```python
from build123d import *

# Parameters (mm, degrees)
SKETCH2_W               = 50.8
SKETCH2_H               = 50.8
BOSS_EXTRUDE1_DEPTH     = 4.7625
SKETCH3_W               = 3.175
SKETCH3_H               = 50.8
CUT_EXTRUDE1_DEPTH      = 1.5875
BOSS_EXTRUDE2_DEPTH     = 6.35
BOSS_EXTRUDE3_DEPTH     = 12.7
SKETCH6_W               = 22.225
SKETCH6_H               = 6.35
CUT_EXTRUDE2_DEPTH      = 44.45
SKETCH7_R               = 2.413
SKETCH7_R_2             = 2.286
CUT_EXTRUDE3_DEPTH      = 50.8
CUT_EXTRUDE4_DEPTH      = 3.175
CUT_EXTRUDE4_DEPTH_BACK = 3.175
SKETCH8_R               = 7.9375


with BuildPart() as part:
    # Sketch2 → Boss-Extrude1 (new body)
    with BuildSketch(Plane(origin=(0, 0, 0), x_dir=(1, 0, 0), z_dir=(0, 1, 0))):
        with Locations((25.4, 25.4)):
            Rectangle(SKETCH2_W, SKETCH2_H)
    extrude(amount=BOSS_EXTRUDE1_DEPTH)

    # Sketch3 → Cut-Extrude1 (cut)
    with BuildSketch(Plane(origin=(0, 4.7625, 0), x_dir=(1, 0, 0), z_dir=(0, 1, 0))):
        with Locations((11.1125, 25.4)):
            Rectangle(SKETCH3_W, SKETCH3_H)
        with Locations((39.6875, 25.4)):
            Rectangle(SKETCH3_W, SKETCH3_H)
    extrude(amount=-CUT_EXTRUDE1_DEPTH, mode=Mode.SUBTRACT)

    # Sketch4 → Boss-Extrude2 (add)
    with BuildSketch(Plane.XY):
        Polygon((50.8, 0), (25.4, 0), (25.4, -31.75), align=None)
        Polygon((25.4, 0), (0, 0), (25.4, -31.75), align=None)
    extrude(amount=-BOSS_EXTRUDE2_DEPTH)

    # Sketch5 → Boss-Extrude3 (add)
    with BuildSketch(Plane(origin=(0, 0, -50.8), x_dir=(-1, 0, 0), z_dir=(0, 0, -1))):
        Polygon((-25.4, 0), (-50.8, 0), (-25.4, -31.75), align=None)
        Polygon((0, 0), (-25.4, 0), (-25.4, -31.75), align=None)
    extrude(amount=-BOSS_EXTRUDE3_DEPTH)

    # Sketch6 → Cut-Extrude2 (cut)
    with BuildSketch(Plane(origin=(0, 4.7625, 0), x_dir=(1, 0, 0), z_dir=(0, 1, 0))):
        with Locations((25.4, 47.625)):
            Rectangle(SKETCH6_W, SKETCH6_H)
    extrude(amount=-CUT_EXTRUDE2_DEPTH, mode=Mode.SUBTRACT)

    # Sketch7 → Cut-Extrude3 (cut)
    with BuildSketch(Plane(origin=(0, 0, -44.45), x_dir=(-1, 0, 0), z_dir=(0, 0, -1))):
        with Locations((-25.4, -26.9875)):
            Circle(SKETCH7_R)
        with Locations((-25.4, -1.5875)):
            Circle(SKETCH7_R_2)
    extrude(amount=-CUT_EXTRUDE3_DEPTH, mode=Mode.SUBTRACT)

    # Sketch8 → Cut-Extrude4 (cut, two sides: drawn at the far end of the back side and taken through both)
    with BuildSketch(Plane.XY.offset(-38.1).offset(-CUT_EXTRUDE4_DEPTH_BACK)):
        with Locations((25.4, -1.5875)):
            Circle(SKETCH8_R)
    extrude(amount=CUT_EXTRUDE4_DEPTH + CUT_EXTRUDE4_DEPTH_BACK, mode=Mode.SUBTRACT)


solid = part.part
```
Check sheet for the modelled part. Datum: model origin and axes. Units: mm. A direction names the side the tool comes from. Coordinates: 2 decimals unless noted, no trailing zeros. Loops run counter-clockwise (first coordinate to the right, second up) from the corner with the lowest first, then second, coordinate; pieces in that order, holes last. Notation, with made-up numbers: M 55,-36 L 73,-36 A20 cw 73,-32 Z; hole C -27.75,54 d5. An arc over 180 degrees is marked long. Answer as a JSON object with one key per item and string values.
1. Release check for a two-part mould opening along X. For faces 5 (the cylindrical face through (27.18, -25.36, -41.32)), 6 (the flat face through (25, 2, -34.925)), 7 (the flat face through (0, 2, -25)), 8 (the flat face through (26, -12, -38.1)) record: pulls with the +X half, pulls with the -X half, needs draft (parallel to the pull), parting line crosses it, or undercut.
Outcome:
{"face 5": "undercut", "face 6": "undercut", "face 7": "pulls with the -X half", "face 8": "needs draft"}
2. Sectioned sample at C-C on z = -13. Record the cut outline in (x, y) (1 decimal), and give its area (3 significant figures).
Outcome:
{"outline": "M 0,0 L 23.8,0 A2.3 cw 27,0 L 50.8,0 L 50.8,4.8 L 41.3,4.8 L 41.3,3.2 L 38.1,3.2 L 38.1,4.8 L 12.7,4.8 L 12.7,3.2 L 9.5,3.2 L 9.5,4.8 L 0,4.8 Z", "area": "230 mm²"}
3. Sectioned sample at A-A on z = -46.5. Record the cut outline in (x, y) (1 decimal), and give its area (3 significant figures).
Outcome:
{"outline": "M 0,0 L 14.3,-17.9 L 14.3,4.8 L 12.7,4.8 L 12.7,3.2 L 9.5,3.2 L 9.5,4.8 L 0,4.8 Z; M 36.5,-17.9 L 50.8,0 L 50.8,4.8 L 41.3,4.8 L 41.3,3.2 L 38.1,3.2 L 38.1,4.8 L 36.5,4.8 Z", "area": "381 mm²"}
4. Depth check by flat-ended pin: P1, Ø5, axis at x = 22.5, y = 2.5, coming from the -Z side; P2, Ø1, axis at x = 10.5, z = -38, coming from the +Y side (3 decimals); P3, Ø3, axis at y = -4, z = -47, coming from the -X side. Enter the tip coordinate at first touch or a pass-through.
Outcome:
{"P1": "z = -44.45", "P2": "y = 3.175", "P3": "x = 2"}
5. Access from +Z, -Z, +X, -X, +Y, -Y to the whole of each face (thin tool, end or side, straight path). Record for faces 1 (the flat face through (36.512, -6, -48)), 2 (the flat face through (39, 0, -22)), 3 (the flat face through (41.275, 4, -25)), 4 (the flat face through (27, -4, -41.275)).
Outcome:
{"face 1": "-Z, +Y, -Y", "face 2": "+X, -X, -Y", "face 3": "+Z, -Z, +Y", "face 4": "none"}
6. Sectioned sample at D-D on z = -4.5. Count the separate pieces of the cut face and the enclosed holes in it, and give its area (3 significant figures).
Outcome:
{"separate pieces": "1", "enclosed holes": "2", "area": "1,000 mm²"}
7. Sectioned sample at B-B on x = 5. Record the cut outline in (y, z).
Outcome:
{"outline": "M -6.25,-50.8 L 4.76,-50.8 L 4.76,0 L -6.25,0 L -6.25,-6.35 L 0,-6.35 L 0,-38.1 L -6.25,-38.1 Z"}
8. Scan lines: L1, parallel to Z at x = 22, y = -10.5; L2, parallel to Z at x = 44, y = -8; L3, parallel to Y at x = 14.5, z = -34. Record each from-to range of solid material in increasing order. Write a range as from..to.
Outcome:
{"L1": "-44.45..-38.1, -6.35..0", "L2": "-50.8..-38.1, -6.35..0", "L3": "0..4.76"}
